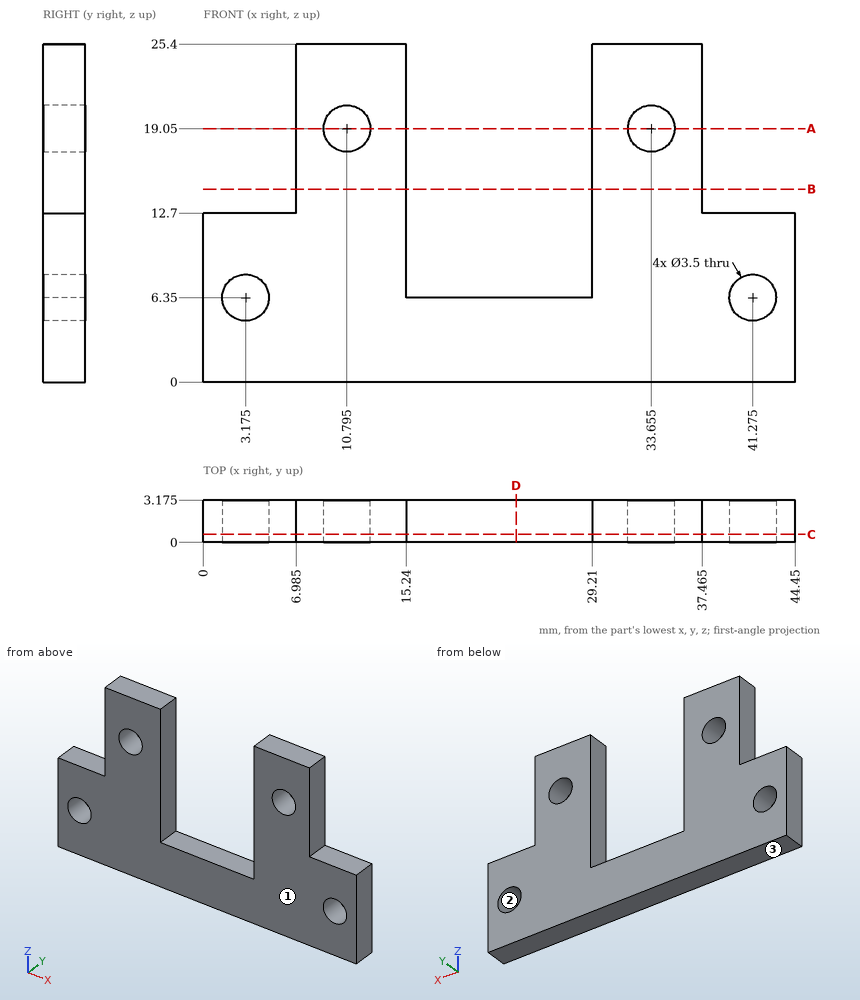
Drawing for the job (mm, zero at the part's lowest x, y, z). Round coordinates to 2 decimals unless told otherwise and drop trailing zeros. Loops run counter-clockwise (first coordinate to the right, second up) from the corner with the lowest first, then second, coordinate; pieces in that order, holes last. Notation, with made-up numbers: (-21, 85) - (35, 85) arc R27 ccw to (35, 110) - close; hole circle Ø6 at (-3, 35.5). An arc over 180 degrees is marked (long way). Return JSON: item names as keys, results as strings. Group by question number.
Q1. Band-saw the part on B-B on z = 14.5. Give the cut face in (x, y) (3 decimals), plus the area to 3 significant figures.
Q2. Drill centre lines: line 1 along X through (y, z) = (1.1, 19.05) (3 decimals); line 2 along X through (y, z) = (1.5, 8.75); line 3 along X through (y, z) = (1.65, 24.25) (3 decimals). Where is each one in solid material? Low to high. Write a range as [from, to].
Q3. Band-saw the part on D-D on x = 23.5. Give the cut face in (y, z) (3 decimals).
Q4. Flat gauge pins, fed straight in: pin 1 Ø1.6 at (x, y) = (40, 2) entering from +Z; pin 2 Ø4.5 at (x, z) = (33.655, 19.05) entering from -Y; pin 3 Ø1 at (y, z) = (1.5, 21.5) entering from -X (3 decimals). Where does each tip first touch, or does it go through?
Q5. Band-saw the part on C-C on y = 0.6. Give the cut face in (x, z) (3 decimals).
Q6. Two-plate mould, pull along Z, no slides. Class the marked faces 1, 2 and 3: +Z half, -Z half, draft (parallel to the pull), parting line (faces both ways), or undercut.
Q7. Band-saw the part on A-A on z = 19.05. Give the cut face in (x, y) (3 decimals).
Solutions:
{
 "1": {"outline": "(6.985, 0) - (15.24, 0) - (15.24, 3.175) - (6.985, 3.175) - close; (29.21, 0) - (37.465, 0) - (37.465, 3.175) - (29.21, 3.175) - close", "area": "52.4 mm^2"},
 "2": {"line 1": "x = [6.985, 9.045], [12.545, 15.24], [29.21, 31.905], [35.405, 37.465]", "line 2": "x = [0, 15.24], [29.21, 44.45]", "line 3": "x = [6.985, 15.24], [29.21, 37.465]"},
 "3": {"outline": "(0, 0) - (3.175, 0) - (3.175, 6.35) - (0, 6.35) - close"},
 "4": {"pin 1": "stops at z = 12.7", "pin 2": "stops at y = 0", "pin 3": "stops at x = 6.985"},
 "5": {"outline": "(0, 0) - (44.45, 0) - (44.45, 12.7) - (37.465, 12.7) - (37.465, 25.4) - (29.21, 25.4) - (29.21, 6.35) - (15.24, 6.35) - (15.24, 25.4) - (6.985, 25.4) - (6.985, 12.7) - (0, 12.7) - close; hole circle Ø3.5 at (3.175, 6.35); hole circle Ø3.5 at (10.795, 19.05); hole circle Ø3.5 at (33.655, 19.05); hole circle Ø3.5 at (41.275, 6.35)"},
 "6": {"face 1": "draft", "face 2": "undercut", "face 3": "-Z half"},
 "7": {"outline": "(6.985, 0) - (9.045, 0) - (9.045, 3.175) - (6.985, 3.175) - close; (12.545, 0) - (15.24, 0) - (15.24, 3.175) - (12.545, 3.175) - close; (29.21, 0) - (31.905, 0) - (31.905, 3.175) - (29.21, 3.175) - close; (35.405, 0) - (37.465, 0) - (37.465, 3.175) - (35.405, 3.175) - close"}
}
